Verification items for the finished model (mm, model axes). A direction names the side the tool comes from. Give positions to 0.01 mm unless a question says otherwise; leave off trailing zeros. Order: outer loops, then holes, each group sorted by start corner. A loop starts at its lowest first (then second) coordinate and runs counter-clockwise, first axis right, second up. Notation, with made-up numbers: (82.25, 88.25) -> (100.25, 88.25) arc R31 ccw to (100.25, 122.25) -> close; hole circle Ø1 at (17.25, 75.5). An arc over 180 degrees is marked (long way). One line per question, with ' | ' between items. Start each with the question number.
Q1. Section check B-B on x = 21. Record the cut outline in (y, z), plus the area to 4 significant figures.
Q2. Section check C-C on y = 6.35. Record the cut outline in (x, z), plus the area to 3 significant figures.
Q3. Section check A-A on x = 14.5. Record the cut outline in (y, z).
Q4. Section check D-D on x = -4. Record the cut outline in (y, z).
Q5. Material ranges on probe 1 along Y at (x, z) = (14.5, -56.3); probe 2 along X at (y, z) = (-13, -33.5), recorded low to high. Write a range as [from, to].
Q6. Access from +Z, -Z, +X, -X, +Y, -Y to the whole of each face (thin tool, end or side, straight path). Record for faces 1 (the flat face through (0, -5, -27)), 2 (the cylindrical face through (-18.253, 6.471, -2.465)), 3 (the flat face through (-24.35, 5, -10)).
Q7. Mould release check, pull along Y, two halves, no side actions. Record for faces 4 (the cylindrical face through (-12.473, -12.141, -57.035)), 5 (the flat face through (24.35, 5, -10)), 6 (the cylindrical face through (12.473, -12.141, -57.035)), 7 (the flat face through (0, 12.7, -3)): released by +Y, released by -Y, zero draft, split by the parting line, or undercut.
Q8. Go/stop test with flat-tipped pins: pin 1 (14.5 mm diameter, centred on x = -4.5, y = -42.5, fed in from +Z); pin 2 (3 mm diameter, centred on x = 14, z = -46, fed in from +Y); pin 3 (24.5 mm diameter, centred on x = 12, z = -19.5, fed in from -Y). Record where each tip stops, or that it passes through.
from build123d import *

# Parameters (mm, degrees)
SKETCH013_W  = 27.35
SKETCH013_H  = 12.7
SKETCH013_R  = 2.75
PAD012_DEPTH = 5
PAD013_DEPTH = 5
SKETCH014_W  = 29
SKETCH014_H  = 56
SKETCH014_R  = 2.75
PAD014_DEPTH = 5
PAD015_DEPTH = 5


with BuildPart() as part:
    # Sketch013 → Pad012 (new body)
    with BuildSketch(Plane.XY):
        with Locations((13.675, 6.35)):
            Rectangle(SKETCH013_W, SKETCH013_H)
        with Locations((21, 6.35)):
            Circle(SKETCH013_R, mode=Mode.SUBTRACT)
    pad012 = extrude(amount=-PAD012_DEPTH)

    # Sketch015 → Pad013 (join)
    with BuildSketch(Plane.XZ):
        with BuildLine():
            Line((27.35, 0), (27.35, -40.764007))
            ThreePointArc((27.35, -40.764007), (27.556989, -44.222692), (28.175, -47.632004))
            ThreePointArc((29, -54.5), (28.793011, -51.041315), (28.175, -47.632004))
            Line((29, -59.5), (29, -54.5))
            Line((0, -59.5), (29, -59.5))
            Line((0, 0), (0, -59.5))
            Line((27.35, 0), (0, 0))
        make_face()
    pad013 = extrude(amount=PAD013_DEPTH)

    # Sketch014 → Pad014 (join)
    with BuildSketch(Plane(origin=(0, -56, -59.5), x_dir=(1, 0, 0), z_dir=(0, 0, 1))):
        with Locations((14.5, 28)):
            Rectangle(SKETCH014_W, SKETCH014_H)
        with Locations((14.5, 14)):
            Circle(SKETCH014_R, mode=Mode.SUBTRACT)
        with Locations((14.5, 42)):
            Circle(SKETCH014_R, mode=Mode.SUBTRACT)
    pad014 = extrude(amount=PAD014_DEPTH)

    # Sketch016 → Pad015 (join)
    with BuildSketch(Plane.YZ.offset(24.35)):
        with BuildLine():
            Line((-56, -54.5), (-56, -59.5))
            Line((-56, -59.5), (0, -59.5))
            Line((0, -59.5), (0, -17.7))
            ThreePointArc((0, -17.7), (8.980256, -13.980256), (12.7, -5))
            Line((12.7, -5), (12.7, 0))
            Line((12.7, 0), (0, 0))
            Line((0, 0), (-5, 0))
            add(Edge.make_bspline(
                [(-5, 0), (-56, 0), (-56, -54.5)],
                knots=[0, 0, 0, 1.570796, 1.570796, 1.570796], degree=2, weights=[1, 0.707107, 1]))
        make_face()
    pad015 = extrude(amount=PAD015_DEPTH)

    # Mirrored013: Pad012, Pad013, Pad014, Pad015 across Sketch013 V_Axis
    add(pad012.mirror(Plane(origin=(0, 0, 0), x_dir=(0, 0, 1), z_dir=(1, 0, 0))))
    add(pad013.mirror(Plane(origin=(0, 0, 0), x_dir=(0, 0, 1), z_dir=(1, 0, 0))))
    add(pad014.mirror(Plane(origin=(0, 0, 0), x_dir=(0, 0, 1), z_dir=(1, 0, 0))))
    add(pad015.mirror(Plane(origin=(0, 0, 0), x_dir=(0, 0, 1), z_dir=(1, 0, 0))))


solid = part.part
Filled in:
1) outline: (-56, -59.5) -> (0, -59.5) -> (0, -5) -> (3.6, -5) -> (3.6, 0) -> (-5, 0) -> (-5, -54.5) -> (-56, -54.5) -> close; (9.1, -5) -> (12.7, -5) -> (12.7, 0) -> (9.1, 0) -> close | area: 588.5 mm²
2) outline: (-29.35, -16) -> (-24.35, -16) -> (-24.35, -5) -> (-23.75, -5) -> (-23.75, 0) -> (-29.35, 0) -> close; (-18.25, -5) -> (18.25, -5) -> (18.25, 0) -> (-18.25, 0) -> close; (23.75, -5) -> (24.35, -5) -> (24.35, -16) -> (29.35, -16) -> (29.35, 0) -> (23.75, 0) -> close | area: 348 mm²
3) outline: (-56, -59.5) -> (-44.75, -59.5) -> (-44.75, -54.5) -> (-56, -54.5) -> close; (-39.25, -59.5) -> (-16.75, -59.5) -> (-16.75, -54.5) -> (-39.25, -54.5) -> close; (-11.25, -59.5) -> (0, -59.5) -> (0, -5) -> (12.7, -5) -> (12.7, 0) -> (-5, 0) -> (-5, -54.5) -> (-11.25, -54.5) -> close
4) outline: (-56, -59.5) -> (0, -59.5) -> (0, -5) -> (12.7, -5) -> (12.7, 0) -> (-5, 0) -> (-5, -54.5) -> (-56, -54.5) -> close
5) probe 1: [-56, -44.75], [-39.25, -16.75], [-11.25, 0] | probe 2: [-29.35, -24.35], [24.35, 29.35]
6) face 1: +Z, -Y | face 2: +Z, -Z | face 3: -Z, +Y
7) face 4: undercut | face 5: zero draft | face 6: undercut | face 7: released by +Y
8) pin 1: z = -54.5 | pin 2: y = 0 | pin 3: y = -5
